Verification items for the finished model (mm, model axes). A direction names the side the tool comes from. Round coordinates to 2 decimals unless told otherwise and drop trailing zeros. Loops run counter-clockwise (first coordinate to the right, second up) from the corner with the lowest first, then second, coordinate; pieces in that order, holes last. Notation, with made-up numbers: (-12, 24.25) -> (-3, 24.25) arc R4 ccw to (-3, 28.25) -> close; hole circle Ø3 at (43, 59.25). An arc over 180 degrees is marked (long way). Write item = value, one per line.
```python
from build123d import *

# Parameters (mm, degrees)
PAD_DEPTH       = 20
SKETCH001_R     = 2.75
POCKET_DEPTH    = 25.001
SKETCH002_R     = 4.75
POCKET001_DEPTH = 20.001


with BuildPart() as part:
    # Sketch → Pad (new body)
    with BuildSketch(Plane.XY):
        with BuildLine():
            ThreePointArc((14.96663, 0), (0, 14), (-14.96663, 0))
            Line((-25.980762, 0), (-14.96663, 0))
            ThreePointArc((25.980762, 0), (0, 25), (-25.980762, 0))
            Line((14.96663, 0), (25.980762, 0))
        make_face()
    extrude(amount=PAD_DEPTH)

    # Sketch001 (on Face2 of Pad) → Pocket (cut, through all)
    with BuildSketch(Plane.XZ):
        with Locations((-19.25, 10)):
            Circle(SKETCH001_R)
        with Locations((19.25, 10)):
            Circle(SKETCH001_R)
    extrude(amount=-POCKET_DEPTH, mode=Mode.SUBTRACT)

    # Sketch002 (on DatumPlane) → Pocket001 (cut, through all)
    with BuildSketch(Plane.XZ.offset(-5)):
        with Locations((-19.25, 10)):
            Circle(SKETCH002_R)
        Polygon((19.25, 5.092523), (23.5, 7.546261), (23.5, 12.453739), (19.25, 14.907477), (15, 12.453739), (15, 7.546261), align=None)
    extrude(amount=-POCKET001_DEPTH, mode=Mode.SUBTRACT)


solid = part.part
```
(1) Material ranges on probe 1 along X at (y, z) = (9.25, 10); probe 2 along Z at (x, y) = (-19.25, 1.95); probe 3 along X at (y, z) = (11.5, 6.5), recorded low to high. Write a range as from..to.
Filled sheet:
probe_1 = -14.5..-10.95, 10.95..15, 23.5..23.89
probe_2 = 0..7.25, 12.75..20
probe_3 = -22.8..-22.46, -16.04..-8.29, 8.29..16.81, 21.69..22.8
(2) Go/stop test with flat-tipped pins: pin 1 Ø8 at (y, z) = (21.5, 3) entering from +X; pin 2 Ø5 at (x, z) = (-19.5, 8.5) entering from +Y; pin 3 Ø11 at (x, z) = (-19.25, 10) entering from -Y; pin 4 Ø4 at (y, z) = (7.5, 6) entering from +X. Record where each tip stops, or that it passes through.
Filled sheet:
pin_1 = 18.27
pin_2 = 5
pin_3 = 0
pin_4 = 25.17
(3) Sectioned sample at B-B, the plane z = 10. Record the cut outline in (x, y).
Filled sheet:
outline = (-25.98, 0) -> (-22, 0) -> (-22, 5) -> (-24, 5) -> (-24, 9) arc R26 ccw to start; (-16.5, 0) -> (-14.97, 0) arc R15 cw to (14.97, 0) -> (16.5, 0) -> (16.5, 5) -> (15, 5) -> (15, 20.24) arc R26 ccw to (-14.5, 20.58) -> (-14.5, 5) -> (-16.5, 5) -> close; (22, 0) -> (25.98, 0) arc R26 ccw to (23.5, 10.12) -> (23.5, 5) -> (22, 5) -> close
(4) Set-up check for faces 1 (the face through (17.155, 12.512, 13.698)), 2 (the face through (23, 0, 10)): record each of +Z, -Z, +X, -X, +Y, -Y from which the full face is reachable in a straight line by a thin tool's end or side.
Filled sheet:
face_1 = +Y
face_2 = +Z, -Z, +X, -X, -Y
(5) Draft check along X on faces 3 (the face through (0.558, 24.994, 9.86)), 4 (the face through (0, 15, 0)), 5 (the face through (20.933, 9.383, 13.936)). Enter one of: released by +X, released by -X, zero draft, split by the parting line, or undercut.
Filled sheet:
face_3 = split by the parting line
face_4 = zero draft
face_5 = undercut
(6) Sectioned sample at D-D, the plane y = 19. Record the cut outline in (x, z).
Filled sheet:
outline = (-16.61, 0) -> (16.61, 0) -> (16.61, 6.61) -> (15, 7.55) -> (15, 12.45) -> (16.61, 13.39) -> (16.61, 20) -> (-16.61, 20) -> (-16.61, 13.95) arc R4.75 cw to (-16.61, 6.05) -> close
(7) Sectioned sample at A-A, the plane x = -19.25. Record the cut outline in (y, z).
Filled sheet:
outline = (0, 0) -> (16.48, 0) -> (16.48, 5.25) -> (5, 5.25) -> (5, 7.25) -> (0, 7.25) -> close; (0, 12.75) -> (5, 12.75) -> (5, 14.75) -> (16.48, 14.75) -> (16.48, 20) -> (0, 20) -> close
(8) Sectioned sample at C-C, the plane y = 6. Record the cut outline in (x, z).
Filled sheet:
outline = (-25.04, 0) -> (-13.27, 0) -> (-13.27, 20) -> (-25.04, 20) -> close; (13.27, 0) -> (25.04, 0) -> (25.04, 20) -> (13.27, 20) -> close; hole circle Ø9.5 at (-19.25, 10); hole (15, 7.55) -> (19.25, 5.09) -> (23.5, 7.55) -> (23.5, 12.45) -> (19.25, 14.91) -> (15, 12.45) -> close
